CAD build for the part. Positions are in the model's coordinates, mm. A direction names the side the tool comes from. Coordinates: 2 decimals unless noted, no trailing zeros. Loops run counter-clockwise (first coordinate to the right, second up) from the corner with the lowest first, then second, coordinate; pieces in that order, holes last. Notation, with made-up numbers: (-39.5, -21) -> (-15.5, -21) arc R15 cw to (-15.5, 5) -> close; hole circle Ø6 at (-31, 15). An arc over 180 degrees is marked (long way). Write each question's results on one line, items separated by ' | '.
Autodesk Inventor part; units mm, degrees
ref_plane "YZ Plane" through (0, 0, 0) normal (1, 0, 0) x (0, 1, 0)
ref_plane "XZ Plane" through (0, 0, 0) normal (0, 1, 0) x (-1, 0, 0)
ref_plane "XY Plane" through (0, 0, 0) normal (0, 0, 1) x (1, 0, 0)
sketch "Sketch1" plane through (0, 0, 0) normal (0, 1, 0) x (-1, 0, 0)
  line L0 (12.5, 12.5) -> (-12.5, 12.5)
  line L1 (-12.5, 12.5) -> (-12.5, -12.5)
  line L2 (-12.5, -12.5) -> (12.5, -12.5)
  line L3 (12.5, -12.5) -> (12.5, 12.5)
  line L4 (12.5, 12.5) -> (-12.5, -12.5) construction
  line L5 (-12.5, 12.5) -> (12.5, -12.5) construction
  point P0 (0, 0)
  dimension "d0" = 25
  dimension "d1" = 25
extrude "Extrusion1" add sketch "Sketch1" along normal blind 12.5
sketch "Sketch2" plane through (0, 12.5, 0) normal (0, 1, 0) x (1, 0, 0)
  line L0 (-12.5, 12.5) -> (-12.5, -12.5) construction
  line L1 (-12.5, 0) -> (12.5, 0) construction
  line L2 (12.5, -12.5) -> (12.5, 12.5) construction
  line L3 (-6.1256, -2.4906) -> (-10.5058, -0.671)
  line L4 (-10.5058, -0.671) -> (-10.5058, 0.0782)
  line L5 (-10.5058, 0.0782) -> (-6.1256, 1.8978)
  line L6 (-6.1256, 1.8978) -> (-6.1256, 0.9551)
  line L7 (-6.1256, 0.9551) -> (-9.1885, -0.3005)
  line L8 (-9.1885, -0.3005) -> (-6.1256, -1.5479)
  line L9 (-6.1256, -1.5479) -> (-6.1256, -2.4906)
  line L10 (-2.7705, -0.7698) -> (-5.0306, -0.7698)
  line L11 (-5.0306, -0.7698) -> (-5.0306, 0.177)
  line L12 (-5.0306, 0.177) -> (-2.7705, 0.177)
  line L13 (-2.7705, 0.177) -> (-2.7705, -0.7698)
  line L14 (2.433, -2.54) -> (0.9592, -2.54)
  line L15 (0.9592, -2.54) -> (-0.0206, -0.9221)
  line L16 (-0.0206, -0.9221) -> (-1.0209, -2.54)
  line L17 (-1.0209, -2.54) -> (-2.433, -2.54)
  line L18 (-2.433, -2.54) -> (-0.7822, 0.0165)
  line L19 (-0.7822, 0.0165) -> (-2.3671, 2.54)
  line L20 (-2.3671, 2.54) -> (-0.8933, 2.54)
  line L21 (-0.8933, 2.54) -> (0.0247, 1.0045)
  line L22 (0.0247, 1.0045) -> (0.9674, 2.54)
  line L23 (0.9674, 2.54) -> (2.3794, 2.54)
  line L24 (2.3794, 2.54) -> (0.7863, 0.07)
  line L25 (0.7863, 0.07) -> (2.433, -2.54)
  line L26 (5.1088, -0.7698) -> (2.8488, -0.7698)
  line L27 (2.8488, -0.7698) -> (2.8488, 0.177)
  line L28 (2.8488, 0.177) -> (5.1088, 0.177)
  line L29 (5.1088, 0.177) -> (5.1088, -0.7698)
  line L30 (10.5881, -0.671) -> (6.208, -2.4906)
  line L31 (6.208, -2.4906) -> (6.208, -1.5479)
  line L32 (6.208, -1.5479) -> (9.2667, -0.2964)
  line L33 (9.2667, -0.2964) -> (6.208, 0.9551)
  line L34 (6.208, 0.9551) -> (6.208, 1.8978)
  line L35 (6.208, 1.8978) -> (10.5881, 0.0782)
  line L36 (10.5881, 0.0782) -> (10.5881, -0.671)
  point P0 (0, 0)
extrude "Extrusion2" cut sketch "Sketch2" against normal blind 5.08
sketch "Sketch3" plane through (-12.5, 0, 12.5) normal (0, 0, 1) x (1, 0, 0)
  line L0 (12.4794, 12.5) -> (11.4791, 12.5) construction
  line L1 (12.5, 0) -> (12.4794, 12.5) construction
  line L2 (11.7157, 8.8011) -> (11.712, 11.0611)
  line L3 (11.712, 11.0611) -> (12.6588, 11.0627)
  line L4 (12.6588, 11.0627) -> (12.6625, 8.8026)
  line L5 (12.6625, 8.8026) -> (11.7157, 8.8011)
  line L6 (9.9531, 4.2081) -> (9.9464, 8.2342)
  line L7 (9.9464, 8.2342) -> (10.8974, 8.2357)
  line L8 (10.8974, 8.2357) -> (14.0629, 5.8986)
  line L9 (14.0629, 5.8986) -> (14.0592, 8.1174)
  line L10 (14.0592, 8.1174) -> (15.0266, 8.119)
  line L11 (15.0266, 8.119) -> (15.0328, 4.3523)
  line L12 (15.0328, 4.3523) -> (14.0654, 4.3507)
  line L13 (14.0654, 4.3507) -> (10.9164, 6.6797)
  line L14 (10.9164, 6.6797) -> (10.9205, 4.2096)
  line L15 (10.9205, 4.2096) -> (9.9531, 4.2081)
  line L16 (11.7278, 1.4404) -> (11.7241, 3.7005)
  line L17 (11.7241, 3.7005) -> (12.6709, 3.7021)
  line L18 (12.6709, 3.7021) -> (12.6746, 1.442)
  line L19 (12.6746, 1.442) -> (11.7278, 1.4404)
extrude "Extrusion3" cut sketch "Sketch3" against normal blind 5.08
sketch "Sketch11" plane through (0, 12.5, 0) normal (0, 1, 0) x (1, 0, 0)
  circle A0 centre (-0.2, 6.5) radius 3
  circle A1 centre (0.2, -6.5) radius 3
  line L0 (12.5, 12.5) -> (-12.5, 12.5)
  line L1 (-12.5, -12.5) -> (12.5, -12.5)
  point P0 (0, 0)
  dimension "d81" = 6
  dimension "d82" = 6
  dimension "d83" = 6
extrude "Extrusion4" cut sketch "Sketch11" against normal blind 25.4
equation "\"d46\" = 0.125 * Sketch7_Pitch"
equation "\"Sketch7_Pitch\" = 1.27"
equation "\"d48\" = 60deg"
equation "\"d67\" = 0.125 * Sketch9_Pitch"
equation "\"Sketch9_Pitch\" = 1.27"
equation "\"d69\" = 60deg"
equation "\"d99\" = 0.125 * Sketch12_Pitch"
equation "\"Sketch12_Pitch\" = 1.27"
equation "\"d101\" = 60deg"
equation "\"d120\" = 0.125 * Sketch14_Pitch"
equation "\"Sketch14_Pitch\" = 1.27"
equation "\"d122\" = 60deg"
equation "\"d143\" = 55deg"
equation "\"Sketch16_Pitch\" = 1.27"
equation "\"d161\" = 55deg"
equation "\"Sketch18_Pitch\" = 1.27"
properties part number "squareCalibrationBlock-25mm"
1) Which spindle directions (+Z, -Z, +X, -X, +Y, -Y) get a long thin tool onto all of the face, cutting with end or side? Do faces 1 (the flat face through (12.5, 6, 0)), 2 (the flat face through (-4, 10, 0.77)). Say none if no direction does.
Outcome:
face 1: +Z, -Z, +X, +Y, -Y | face 2: +Y
2) Slice it at A-A (z = -6.5). Write the cut outline in (x, y), then the cut area to 4 significant figures.
Outcome:
outline: (-12.5, 0) -> (-3.2, 0) -> (-3.2, 12.5) -> (-12.5, 12.5) -> close; (2.8, 0) -> (12.5, 0) -> (12.5, 12.5) -> (2.8, 12.5) -> close | area: 237.5 mm^2
3) Slice it at C-C (x = -6.5). Write the cut outline in (y, z).
Outcome:
outline: (0, -12.5) -> (12.5, -12.5) -> (12.5, -1.74) -> (7.42, -1.74) -> (7.42, -0.8) -> (12.5, -0.8) -> (12.5, 1.4) -> (7.42, 1.4) -> (7.42, 2.34) -> (12.5, 2.34) -> (12.5, 12.5) -> (0, 12.5) -> close
4) Slice it at B-B (x = 8). Write the cut outline in (y, z), then the cut area to 3 significant figures.
Outcome:
outline: (0, -12.5) -> (12.5, -12.5) -> (12.5, -1.15) -> (7.42, -1.15) -> (7.42, -0.22) -> (12.5, -0.22) -> (12.5, 0.81) -> (7.42, 0.81) -> (7.42, 1.75) -> (12.5, 1.75) -> (12.5, 12.5) -> (0, 12.5) -> close | area: 303 mm^2
5) Pin check, flat tip, straight feed: pin 1 (10 mm diameter, centred on x = -5, z = -1.5, fed in from -Y). Stop position of the tip, or through.
Outcome:
pin 1: stops at y = 0
6) Drill centre lines: L1, parallel to X at y = 3.75, z = 6.5; L2, parallel to Z at x = -4, y = 9.25; L3, parallel to Z at x = 1.25, y = 7.75. Where is each one in solid material? Low to high. Write a range as from..to.
Outcome:
L1: x = -12.5..-2.8, 3.2..12.5 | L2: z = -12.5..-0.18, 0.77..12.5 | L3: z = -12.5..-9.13, -3.87..-2.54, -0.79..0.66, 2.54..3.69, 9.31..12.5
